Source: CAD feature listing. Evaluate the final solid. Frame: model axes, mm. A direction names the side the tool comes from. Round coordinates to 2 decimals unless told otherwise and drop trailing zeros. Order: outer loops, then holes, each group sorted by start corner. A loop starts at its lowest first (then second) coordinate and runs counter-clockwise, first axis right, second up.
```python
from build123d import *

# Parameters (mm, degrees)
EXTRUDE_1_DEPTH        = 19
CUT_EXTRUDE_1_REACH    = 68.114
EXTRUDE_START          = 97
EXTRUDE_2_DEPTH        = 97
CUT_EXTRUDE_2_REACH    = 134.159
SKETCH_8_R             = 2.1
HOLE_WIZARD_M5_1_D     = 4.2
HOLE_WIZARD_M5_1_DEPTH = 3
HOLE_WIZARD_M5_2_D     = 4.2


with BuildPart() as part:
    # 草图2 → 凸台-拉伸1 (new body)
    with BuildSketch(Plane.XY.offset(-72.500175037)):
        with BuildLine():
            Line((-9.84018, -23), (-11.373653726, -22.694973111))
            Line((-11.373653726, -22.694973111), (-12.673669978, -21.826330022))
            Line((-12.673669978, -21.826330022), (-22.257871236, -12.242128764))
            Line((-22.257871236, -12.242128764), (-23, -10.450471437))
            Line((-23, -10.450471437), (-23, 10.450471437))
            Line((-23, 10.450471437), (-22.257871236, 12.242128764))
            Line((-22.257871236, 12.242128764), (-12.673669978, 21.826330022))
            Line((-12.673669978, 21.826330022), (-11.373653726, 22.694973111))
            Line((-11.373653726, 22.694973111), (-9.84018, 23))
            Line((-9.84018, 23), (36.000000003, 23))
            ThreePointArc((36.000000003, 23), (59.000000003, 0), (36.000000003, -23))
            Line((36.000000003, -23), (-9.84018, -23))
        make_face()
    extrude(amount=EXTRUDE_1_DEPTH)

    # 草图4 → 切除-拉伸1 (cut, up to next)
    with BuildSketch(Plane.XY.offset(-53.500175037), mode=Mode.PRIVATE) as cut_extrude_1_sk1:
        Polygon((5.790000003, -9), (-5.789999997, -9), (-8.999999997, -5.79), (-8.999999997, 5.79), (-5.789999997, 9), (5.790000003, 9), (9.000000003, 5.79), (9.000000003, -5.79), align=None)
    cut_extrude_1_tool1 = extrude(cut_extrude_1_sk1.sketch, amount=-CUT_EXTRUDE_1_REACH, mode=Mode.PRIVATE) & part.part
    add(cut_extrude_1_tool1.solids().sort_by_distance((0, 0, -53.500175))[0], mode=Mode.SUBTRACT)

    # 草图7 → 凸台-拉伸2 (add)
    with BuildSketch(Plane(origin=(0, 0, -72.500175037), x_dir=(-1, 0, 0), z_dir=(0, 0, -1)).offset(EXTRUDE_START)):
        with BuildLine():
            Line((-36.000000003, 23), (9.84018, 23))
            Line((9.84018, 23), (11.373653726, 22.694973111))
            Line((11.373653726, 22.694973111), (12.673669978, 21.826330022))
            Line((12.673669978, 21.826330022), (22.257871236, 12.242128764))
            Line((22.257871236, 12.242128764), (22.628935618, 11.3463001))
            Line((22.628935618, 11.3463001), (23, 10.450471437))
            Line((23, 10.450471437), (23, -10.450471437))
            Line((23, -10.450471437), (22.628935618, -11.3463001))
            Line((22.628935618, -11.3463001), (22.257871236, -12.242128764))
            Line((22.257871236, -12.242128764), (12.673669978, -21.826330022))
            Line((12.673669978, -21.826330022), (11.373653726, -22.694973111))
            Line((11.373653726, -22.694973111), (9.84018, -23))
            Line((9.84018, -23), (-36.000000003, -23))
            ThreePointArc((-36.000000003, -23), (-59, 0), (-36.000000003, 23))
        make_face()
        with BuildLine():
            Line((3.252486509, 20), (8.556678261, 20))
            ThreePointArc((8.556678261, 20), (9.890133674, 19.734759227), (11.020582589, 18.979417411))
            Line((11.020582589, 18.979417411), (19.35467064, 10.64532936))
            ThreePointArc((19.35467064, 10.64532936), (19.832284364, 9.930529909), (20, 9.087366467))
            Line((20, 9.087366467), (20, -9.087366467))
            ThreePointArc((20, -9.087366467), (19.832284364, -9.930529909), (19.35467064, -10.64532936))
            Line((19.35467064, -10.64532936), (11.020582589, -18.979417411))
            ThreePointArc((11.020582589, -18.979417411), (9.890133674, -19.734759227), (8.556678261, -20))
            Line((8.556678261, -20), (-36, -20))
            ThreePointArc((-36, -20), (-56, 0), (-36, 20))
            Line((-36, 20), (3.252486509, 20))
        make_face(mode=Mode.SUBTRACT)
    extrude(amount=-EXTRUDE_2_DEPTH)

    # 草图8 → 切除-拉伸2 (cut, up to next)
    with BuildSketch(Plane.XY.offset(-53.500175037), mode=Mode.PRIVATE) as cut_extrude_2_sk1:
        with Locations((49.800000003, 0)):
            Circle(SKETCH_8_R)
    cut_extrude_2_tool1 = extrude(cut_extrude_2_sk1.sketch, amount=-CUT_EXTRUDE_2_REACH, mode=Mode.PRIVATE) & part.part
    # 草图8 → 切除-拉伸2 (cut, up to next)
    with BuildSketch(Plane.XY.offset(-53.500175037), mode=Mode.PRIVATE) as cut_extrude_2_sk2:
        with Locations((-8.579999997, -15.24)):
            Circle(SKETCH_8_R)
    cut_extrude_2_tool2 = extrude(cut_extrude_2_sk2.sketch, amount=-CUT_EXTRUDE_2_REACH, mode=Mode.PRIVATE) & part.part
    # 草图8 → 切除-拉伸2 (cut, up to next)
    with BuildSketch(Plane.XY.offset(-53.500175037), mode=Mode.PRIVATE) as cut_extrude_2_sk3:
        with Locations((-8.579999997, 15.24)):
            Circle(SKETCH_8_R)
    cut_extrude_2_tool3 = extrude(cut_extrude_2_sk3.sketch, amount=-CUT_EXTRUDE_2_REACH, mode=Mode.PRIVATE) & part.part
    add(cut_extrude_2_tool1.solids().sort_by_distance((49.8, 0, -53.500175))[0], mode=Mode.SUBTRACT)
    add(cut_extrude_2_tool2.solids().sort_by_distance((-8.58, -15.24, -53.500175))[0], mode=Mode.SUBTRACT)
    add(cut_extrude_2_tool3.solids().sort_by_distance((-8.58, 15.24, -53.500175))[0], mode=Mode.SUBTRACT)

    # M5 螺纹孔1
    with Locations(Plane(origin=(0, -23, 0), x_dir=(-1, 0, 0), z_dir=(0, -1, 0))):
        with Locations((-1.619865001, 82.500175037), (-24.539955002, 82.500175037), (-24.539955002, 140.500175037), (-1.619865001, 140.500175037)):
            Hole(HOLE_WIZARD_M5_1_D / 2, depth=HOLE_WIZARD_M5_1_DEPTH)

    # M5 螺纹孔2 (through all)
    with Locations(Plane(origin=(0, 23, 0), x_dir=(1, 0, 0), z_dir=(0, 1, 0))):
        with Locations((24.539955002, 140.500175037), (1.619865001, 140.500175037), (24.539955002, 82.500175037), (1.619865001, 82.500175037)):
            Hole(HOLE_WIZARD_M5_2_D / 2)


solid = part.part
```
1. Pull-direction query (Y, two-part tool) for faces 1 (the face through (-17.4, 17.1, -112.3)), 2 (the face through (24.267, -21.479, -84.582)), 3 (the face through (-17.5, -17, -112.3)), 4 (the face through (7.42, -7.37, -62.87)); classes: released by +Y, released by -Y, zero draft, split by the parting line, or undercut.
2. Section A-A on z = -156. Return loops of the section in (x, y).
3. First-contact query: pin 1 (10 mm diameter, centred on x = 46.5, y = -10, fed in from -Z); pin 2 (10 mm diameter, centred on y = 3.5, z = -98, fed in from +X); pin 3 (12 mm diameter, centred on x = 50.5, z = -122, fed in from +Y). Flat tips, straight axial feed; report the tip coordinate or a pass-through.
4. Access query for faces 5 (the face through (24.813, 21.479, -84.582)), 6 (the face through (-9, 0, -63)), 7 (the face through (56, 0, -122)). Directions: +Z, -Z, +X, -X, +Y, -Y. A direction counts if a zero-diameter tool reaches every point of the face in a straight line with its end or side. Return the directions, or none.
5. Line query: line 1 along X through (y, z) = (-0.5, -121.5); line 2 along Y through (x, z) = (2.5, -154); line 3 along Z through (x, y) = (30.5, -15.5). Output: solid intervals per line, ascending.
6. Section B-B on y = -15.24. Return loops of the section in (x, z), plus the area to 3 significant figures.
7. Section C-C on x = 49.8. Return loops of the section in (y, z), plus the area to 3 significant figures.
8. Section D-D on x = 40. Return loops of the section in (y, z), plus the area to 3 significant figures.
Result:
1. face 1: released by +Y
1. face 2: zero draft
1. face 3: released by -Y
1. face 4: undercut
2. outline: (-23, -10.45) - (-22.26, -12.24) - (-12.67, -21.83) - (-11.37, -22.69) - (-9.84, -23) - (36, -23) arc R23 ccw to (36, 23) - (-9.84, 23) - (-11.37, 22.69) - (-12.67, 21.83) - (-22.26, 12.24) - (-23, 10.45) - close; hole (-20, -9.09) arc R2.2 ccw to (-19.35, -10.65) - (-11.02, -18.98) arc R3.48 ccw to (-8.56, -20) - (36, -20) arc R20 ccw to (36, 20) - (-8.56, 20) arc R3.48 ccw to (-11.02, 18.98) - (-19.35, 10.65) arc R2.2 ccw to (-20, 9.09) - close
3. pin 1: stops at z = -72.5
3. pin 2: stops at x = 59
3. pin 3: stops at y = 21.37
4. face 5: +Y, -Y
4. face 6: +Z, -Z
4. face 7: -Z
5. line 1: x = -23 to -20, 55.99 to 58.99
5. line 2: y = -23 to -20, 20 to 23
5. line 3: z = -72.5 to -53.5
6. outline: (-19.26, -169.5) - (-14.76, -169.5) - (-14.76, -72.5) - (-10.68, -72.5) - (-10.68, -53.5) - (-19.26, -53.5) - close; (-6.48, -72.5) - (48.95, -72.5) - (48.95, -169.5) - (53.23, -169.5) - (53.23, -53.5) - (-6.48, -53.5) - close
6. area: 2,150 mm2
7. outline: (-18.4, -169.5) - (-14.48, -169.5) - (-14.48, -72.5) - (-2.1, -72.5) - (-2.1, -53.5) - (-18.4, -53.5) - close; (2.1, -72.5) - (14.48, -72.5) - (14.48, -169.5) - (18.4, -169.5) - (18.4, -53.5) - (2.1, -53.5) - close
7. area: 1,380 mm2
8. outline: (-22.65, -169.5) - (-19.6, -169.5) - (-19.6, -72.5) - (19.6, -72.5) - (19.6, -169.5) - (22.65, -169.5) - (22.65, -53.5) - (-22.65, -53.5) - close
8. area: 1,450 mm2
